Part model, mm, in its own coordinate system. A direction names the side the tool comes from. Coordinates: 2 decimals unless noted, no trailing zeros. Order: outer loops, then holes, each group sorted by start corner. A loop starts at its lowest first (then second) coordinate and runs counter-clockwise, first axis right, second up. Notation, with made-up numbers: (33.25, 20.5) - (92.25, 20.5) arc R20 cw to (92.25, 30.5) - close; hole circle Ø1 at (36.25, -10). An arc over 180 degrees is marked (long way). Use a Markdown table: item, result. Add a question column.
1) Tool access for faces 4 (the face through (223.873, 242, 1)), 5 (the face through (214.98, 234.44, 1)): list every direction of +Z, -Z, +X, -X, +Y, -Y with a clear straight run to the whole face (end or side of a thin tool).
2) Saw through at C-C on x = 222.5. List the corners of the cut face in (y, z), then the cut area to 3 significant figures.
3) Saw through at D-D on x = 203.5. List the corners of the cut face in (y, z), then the cut area to 3 significant figures.
4) Saw through at A-A on z = 2.05. List the corners of the cut face in (x, y).
5) Wall check: L1, parallel to Y at x = 218.5, z = 2.6; L2, parallel to Y at x = 213.5, z = 2.6; L3, parallel to X at y = 244, z = 0.95. Give the ranges that are in metal, low to high. Write a range as [from, to].
6) Saw through at B-B on y = 232.5. List the corners of the cut face in (x, z).
7) Two-plate mould, pull along X, no slides. Class faces 1 (the face through (216, 239, 0)), 2 (the face through (213.6, 258.31, 1.48)), 3 (the face through (216, 247.702, 2)): +X half, -X half, draft (parallel to the pull), parting line (faces both ways), or undercut.
8) Drop flat-ended pins along their axis: P1, Ø1.5, axis at y = 240.5, z = 1, coming from the -X side; P2, Ø0.6, axis at y = 250, z = 2.5, coming from the -X side; P3, Ø8, axis at x = 210.5, y = 250.5, coming from the -Z side; P4, Ø1.5, axis at y = 241, z = 2, coming from the +X side. Give the stop position or say it passes through.
```python
from build123d import *

# Parameters (mm, degrees)
MODEL_R                 = 16.5
MODEL_R_2               = 2
MODEL_R_3               = 1.5
SALIENTE_EXTRUIR1_DEPTH = 3
CROQUIS2_W              = 6.5
CROQUIS2_H              = 6.5
CROQUIS2_W_2            = 6.500000001
CORTAR_EXTRUIR1_DEPTH   = 2


with BuildPart() as part:
    # Model → Saliente-Extruir1 (new body)
    with BuildSketch(Plane.XY):
        with Locations((215.747807914, 241.952019993)):
            Circle(MODEL_R)
        with Locations((215.747807914, 241.952019993)):
            Circle(MODEL_R_2, mode=Mode.SUBTRACT)
        with Locations((215.747807914, 250.952019993)):
            Circle(MODEL_R_3, mode=Mode.SUBTRACT)
        with Locations((215.747807914, 232.952019993)):
            Circle(MODEL_R_3, mode=Mode.SUBTRACT)
        with BuildLine():
            Line((223.122807913, 245.202019993), (221.372807913, 245.202019993))
            ThreePointArc((221.372807913, 245.202019993), (220.842477828, 244.982350079), (220.622807913, 244.452019993))
            Line((220.622807913, 244.452019993), (220.622807913, 239.452019993))
            ThreePointArc((220.622807913, 239.452019993), (220.842477828, 238.921689907), (221.372807913, 238.702019993))
            Line((221.372807913, 238.702019993), (223.122807913, 238.702019993))
            ThreePointArc((223.122807913, 238.702019993), (223.653137999, 238.921689907), (223.872807913, 239.452019993))
            Line((223.872807913, 239.452019993), (223.872807913, 244.452019993))
            ThreePointArc((223.872807913, 244.452019993), (223.653137999, 244.982350079), (223.122807913, 245.202019993))
        make_face(mode=Mode.SUBTRACT)
        with BuildLine():
            Line((208.372807913, 245.202019993), (210.122807913, 245.202019993))
            ThreePointArc((210.122807913, 245.202019993), (210.653137999, 244.982350079), (210.872807913, 244.452019993))
            Line((210.872807913, 244.452019993), (210.872807913, 239.452019993))
            ThreePointArc((210.872807913, 239.452019993), (210.653137999, 238.921689907), (210.122807913, 238.702019993))
            Line((210.122807913, 238.702019993), (208.372807913, 238.702019993))
            ThreePointArc((208.372807913, 238.702019993), (207.842477828, 238.921689907), (207.622807913, 239.452019993))
            Line((207.622807913, 239.452019993), (207.622807913, 244.452019993))
            ThreePointArc((207.622807913, 244.452019993), (207.842477828, 244.982350079), (208.372807913, 245.202019993))
        make_face(mode=Mode.SUBTRACT)
    extrude(amount=SALIENTE_EXTRUIR1_DEPTH)

    # Croquis2 → Cortar-Extruir1 (cut)
    with BuildSketch(Plane.XY.offset(3)):
        with Locations((215.747807914, 250.952019993)):
            Rectangle(CROQUIS2_W, CROQUIS2_H)
        with Locations((215.747807914, 232.952019993)):
            Rectangle(CROQUIS2_W_2, CROQUIS2_H)
    extrude(amount=-CORTAR_EXTRUIR1_DEPTH, mode=Mode.SUBTRACT)


solid = part.part
```
Results are:
| question | item | result |
|---|---|---|
| 1 | face 4 | +Z, -Z |
| 1 | face 5 | +Z |
| 2 | outline | (226.9, 0) - (238.7, 0) - (238.7, 3) - (226.9, 3) - close; (245.2, 0) - (257.01, 0) - (257.01, 3) - (245.2, 3) - close |
| 2 | area | 70.8 mm2 |
| 3 | outline | (230.9, 0) - (253.01, 0) - (253.01, 3) - (230.9, 3) - close |
| 3 | area | 66.3 mm2 |
| 4 | outline | circle Ø33 at (215.75, 241.95); hole (207.62, 239.45) arc R0.75 ccw to (208.37, 238.7) - (210.12, 238.7) arc R0.75 ccw to (210.87, 239.45) - (210.87, 244.45) arc R0.75 ccw to (210.12, 245.2) - (208.37, 245.2) arc R0.75 ccw to (207.62, 244.45) - close; hole (212.5, 229.7) - (219, 229.7) - (219, 236.2) - (212.5, 236.2) - close; hole (212.5, 247.7) - (219, 247.7) - (219, 254.2) - (212.5, 254.2) - close; hole circle Ø4 at (215.75, 241.95); hole (220.62, 239.45) arc R0.75 ccw to (221.37, 238.7) - (223.12, 238.7) arc R0.75 ccw to (223.87, 239.45) - (223.87, 244.45) arc R0.75 ccw to (223.12, 245.2) - (221.37, 245.2) arc R0.75 ccw to (220.62, 244.45) - close |
| 5 | L1 | [225.68, 229.7], [236.2, 247.7], [254.2, 258.22] |
| 5 | L2 | [225.61, 229.7], [236.2, 247.7], [254.2, 258.3] |
| 5 | L3 | [199.38, 207.62], [210.87, 220.62], [223.87, 232.12] |
| 6 | outline | (202.22, 0) - (214.32, 0) - (214.32, 1) - (212.5, 1) - (212.5, 3) - (202.22, 3) - close; (217.18, 0) - (229.27, 0) - (229.27, 3) - (219, 3) - (219, 1) - (217.18, 1) - close |
| 7 | face 1 | draft |
| 7 | face 2 | parting line |
| 7 | face 3 | undercut |
| 8 | P1 | x = 199.26 |
| 8 | P2 | x = 201.18 |
| 8 | P3 | z = 0 |
| 8 | P4 | x = 232.25 |
